Answer from the drawing. Dimensions are ordinates in mm from the lowest x, y and z of the part. Give positions to 0.01 mm unless a question says otherwise; leave off trailing zeros. Loops run counter-clockwise (first coordinate to the right, second up) from the corner with the lowest first, then second, coordinate; pieces in that order, holes last. Notation, with made-up numbers: (-34, -1) - (-20, -1) arc R29 cw to (-20, 35) - close; hole circle Ø10 at (34.5, -22). An arc over 180 degrees is marked (long way). One line per item, written item: value.
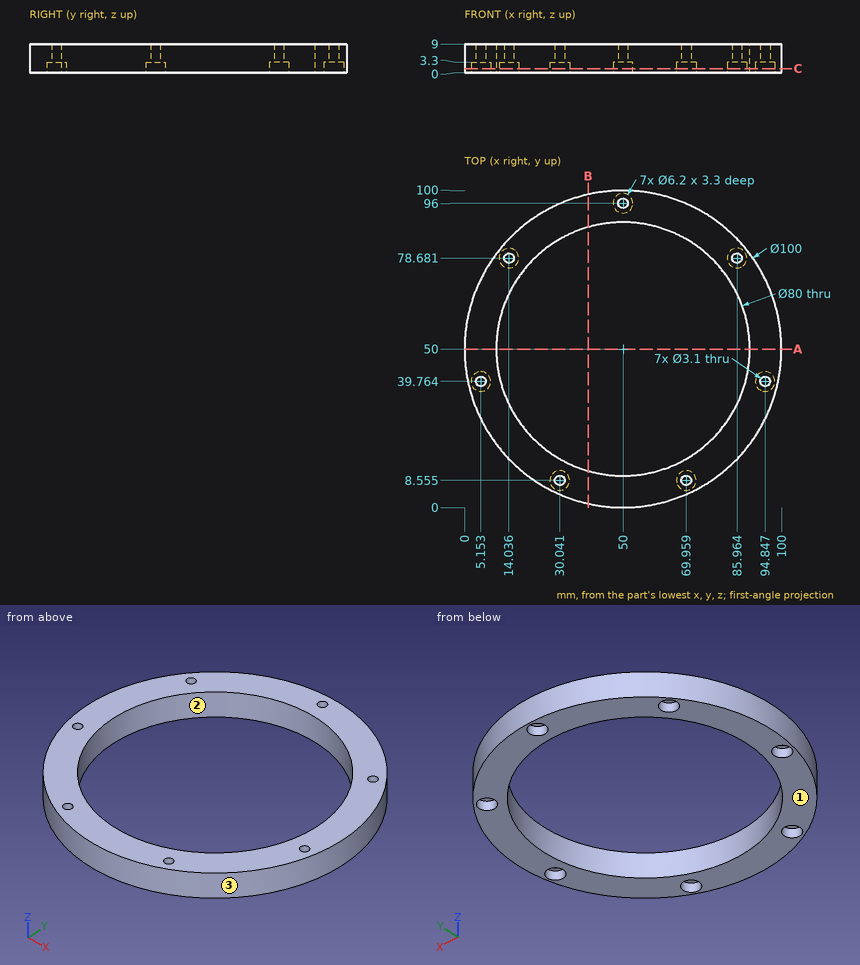
1. Section C-C (z = 1.25) is taken. Count the separate pieces of the cut face and the enclosed holes in it, and give its area (3 significant figures).
Output:
separate pieces: 1
enclosed holes: 8
area: 2,620 mm²
2. The mould has two halves that part along X. Classify the marked faces 1, 2 and 3: released by +X, released by -X, zero draft, split by the parting line, or undercut.
Output:
face 1: zero draft
face 2: undercut
face 3: split by the parting line
3. Flat-ended cylindrical pins translate along their axes: pin 1 Ø1.9 at (x, y) = (70.5, 7.5) entering from -Z; pin 2 Ø4 at (x, z) = (10.5, 5.5) entering from +Y; pin 3 Ø2 at (x, z) = (54, 4.5) entering from -Y. Find the tip coordinate at first contact, or state that the pin passes through.
Output:
pin 1: stops at z = 3.3
pin 2: stops at y = 83.07
pin 3: stops at y = 0.09
4. Section B-B (x = 39) is taken. Write down the section's boundary in (y, z) (1 decimal).
Output:
outline: (1.2, 0) - (11.5, 0) - (11.5, 9) - (1.2, 9) - close; (88.5, 0) - (98.8, 0) - (98.8, 9) - (88.5, 9) - close
5. Section A-A (y = 50) is taken. Write down the section's boundary in (x, z), and give its area (3 significant figures).
Output:
outline: (0, 0) - (10, 0) - (10, 9) - (0, 9) - close; (90, 0) - (100, 0) - (100, 9) - (90, 9) - close
area: 180 mm²
6. Find the intervals of material crossed by line 1 along Y through (x, z) = (50.5, 0.5); line 2 along Y through (x, z) = (70.5, 7) (1 decimal); line 3 along X through (y, z) = (52, 5.5), in increasing order.
Output:
line 1: y = 0 to 10, 90 to 92.94, 99.06 to 100
line 2: y = 4.4 to 7.1, 10 to 15.7, 84.3 to 95.6
line 3: x = 0.04 to 10.05, 89.95 to 99.96
